Autodesk Fusion 360 part; units mm, degrees
sketch "Sketch1" plane through (0, 0, 0) normal (0, 0, 1) x (1, 0, 0)
  line L0 (284.2, -291.299) -> (-284.2, -291.299)
  line L1 (-284.2, -291.299) -> (-284.2, 291.299)
  line L2 (-284.2, 291.299) -> (284.2, 291.299)
  line L3 (284.2, 291.299) -> (284.2, -291.299)
  line L4 (284.2, -291.299) -> (-284.2, 291.299) construction
  line L5 (-284.2, -291.299) -> (284.2, 291.299) construction
  line L6 (-261.35, 291.299) -> (-261.35, -291.299) construction
  circle A0 centre (-261.35, 280.639) radius 2
  circle A1 centre (-261.35, 266.5) radius 2
  circle A2 centre (-261.35, -280.639) radius 2
  circle A3 centre (-261.35, -266.5) radius 2
  line L7 (261.35, 291.299) -> (261.35, -291.299) construction
  circle A4 centre (261.35, 280.639) radius 2
  circle A5 centre (261.35, 266.5) radius 2
  circle A6 centre (261.35, -280.639) radius 2
  circle A7 centre (261.35, -266.5) radius 2
  line L8 (-261.35, -266.5) -> (261.35, -266.5) construction
  circle A8 centre (0, -273.16) radius 2
  line L9 (0, -291.299) -> (0, 291.299) construction
  circle A9 centre (0, 273.16) radius 2
  circle A10 centre (0, 287.299) radius 2
  circle A11 centre (0, -287.299) radius 2
  line L10 (200, 225) -> (-200, 225)
  line L11 (-200, 225) -> (-200, -225)
  line L12 (-200, -225) -> (200, -225)
  line L13 (200, -225) -> (200, 225)
  line L14 (200, 225) -> (-200, -225) construction
  line L15 (-200, 225) -> (200, -225) construction
  line L16 (-289.2, 296.299) -> (289.2, 296.299)
  line L17 (289.2, 296.299) -> (289.2, -296.299)
  line L18 (289.2, -296.299) -> (-289.2, -296.299)
  line L19 (-289.2, -296.299) -> (-289.2, 296.299)
  circle A12 centre (279.2, 101.299) radius 2
  circle A13 centre (279.2, -101.299) radius 2
  circle A14 centre (-279.2, -101.299) radius 2
  circle A15 centre (-279.2, 101.299) radius 2
  line L20 (-304.8, -372.499) -> (304.8, -372.499) construction
  line L21 (304.8, -372.499) -> (304.8, 541.901) construction
  line L22 (304.8, 541.901) -> (-304.8, 541.901) construction
  line L23 (-304.8, 541.901) -> (-304.8, -372.499) construction
  line L24 (0, -372.499) -> (0, -296.299) construction
  line L25 (-261.35, 266.5) -> (261.35, 266.5) construction
  line L26 (261.35, -280.639) -> (-261.35, -280.639) construction
  line L27 (261.35, 280.639) -> (-261.35, 280.639) construction
  dimension "d1" = 568.4
  dimension "d2" = 582.598
  dimension "d3" = 22.85
  dimension "d4" = 4
  dimension "d6" = 4
  dimension "d8" = 4
  dimension "d9" = 4
  dimension "d12" = 22.85
  dimension "d13" = 4
  dimension "d14" = 4
  dimension "d17" = 4
  dimension "d18" = 4
  dimension "d21" = 4
  dimension "d22" = 4
  dimension "d23" = 4
  dimension "d24" = 4
  dimension "d28" = 450
  dimension "d29" = 400
  dimension "d30" = 5
  dimension "d31" = 5
  dimension "d32" = 5
  dimension "d33" = 5
  dimension "d37" = 4
  dimension "d38" = 4
  dimension "d39" = 4
  dimension "d40" = 4
  dimension "d41" = 190
  dimension "d42" = 190
  dimension "d43" = 5
  dimension "d44" = 5
  dimension "d45" = 190
  dimension "d46" = 190
  dimension "d47" = 5
  dimension "d49" = 5
  dimension "d51" = 609.6
  dimension "d52" = 76.2
  dimension "d53" = 914.4
  dimension "d54" = 24.799
  dimension "d55" = 24.799
  dimension "d56" = 10.66
  dimension "d57" = 10.66
  dimension "d61" = 4
  dimension "d62" = 14.139
  dimension "d63" = 14.139
  dimension "d64" = 4
extrude "Extrude1" add sketch "Sketch1" along normal blind 5 contours L0 L1 L2 L3 | L16 L17 L18 L19 makes body 1
fillet "Fillet1" radius 20 4 edges at (-200, -225, 2.5) (200, -225, 2.5) (200, 225, 2.5) (-200, 225, 2.5) on bodies 1
copy_body "Body->Comp1" bodies 1 removing the originals makes body 2 in component "Front Panel"
component "Front Panel" placed x (1, 0, 0) y (0, 1, 0) z (0, 0, 1) at (0, 0, 0)
equation "d1 = XRailLength + 218.4 mm"
equation "d2 = PrintHeight + 282.598 mm"
equation "d28 = PrintHeight + 150 mm"
equation "d29 = XRailLength + 50 mm"
equation "d30 = WallThickness"
equation "d31 = WallThickness"
equation "d32 = WallThickness"
equation "d33 = WallThickness"
equation "WallThickness = 5 mm"
equation "XRailLength = 350 mm"
equation "PrintHeight = 300 mm"
For this review, take the finished solid that the model builds, in its own axes (mm). A direction names the side the tool comes from. Give positions to 0.01 mm unless a question says otherwise; leave off trailing zeros. Order: outer loops, then holes, each group sorted by start corner. A loop starts at its lowest first (then second) coordinate and runs counter-clockwise, first axis right, second up. Notation, with made-up numbers: M 3.25,34 L 36.25,34 A16 ccw 36.25,38 Z; hole C -23.75,81.25 d9. An arc over 180 degrees is marked long. Answer in a Markdown table with one row per item. Add a question column.
(1) For faces 1 (the face through (253, 4, 0)), 2 (the face through (-193.986, 219.297, 2.535)), list the 3-axis set-ups (+Z, -Z, +X, -X, +Y, -Y) from which the entire face can be reached by the end or side of a thin tool; tool diameter is ignored.
(2) For pin 1 (3.5 mm diameter, centred on x = 0, y = 273.16, fed in from +Z), flat-tipped, find the tip position at first contact; note if it passes through.
(3) Wall thickness on probe 1 along Y at (x, z) = (0, 4.05); probe 2 along Y at (x, z) = (261.35, 3.8); probe 3 along X at (y, z) = (-266.5, 1.3): over which ranges is each line inside the solid? List them lowest first. Write a range as [from, to].
(4) Consider section C-C on z = 1.8. Give the number of separate pieces and of enclosed holes in the cut face, and give its area (3 significant figures).
(5) Mouldability with a two-part tool opening along Y and no side actions: class faces 3 (the face through (193.986, -219.297, 2.535)), 4 (the face through (253, 4, 5)) as +Y half, -Y half, draft (parallel to the pull), parting line (faces both ways), or undercut.
(6) Consider section A-A on y = 58.5. State the section outline as (x, z) points, and give its area (3 significant figures).
(7) Consider section B-B on x = 44. State the section outline as (y, z) points.
Evaluation:
| question | item | result |
|---|---|---|
| 1 | face 1 | -Z, +X, -X, +Y, -Y |
| 1 | face 2 | +Z, -Z |
| 2 | pin 1 | passes through |
| 3 | probe 1 | y = [-296.3, -289.3], [-285.3, -275.16], [-271.16, -225], [225, 271.16], [275.16, 285.3], [289.3, 296.3] |
| 3 | probe 2 | y = [-296.3, -282.64], [-278.64, -268.5], [-264.5, 264.5], [268.5, 278.64], [282.64, 296.3] |
| 3 | probe 3 | x = [-289.2, -263.35], [-259.35, 259.35], [263.35, 289.2] |
| 4 | separate pieces | 1 |
| 4 | enclosed holes | 17 |
| 4 | area | 163,000 mm^2 |
| 5 | face 3 | undercut |
| 5 | face 4 | draft |
| 6 | outline | M -289.2,0 L -200,0 L -200,5 L -289.2,5 Z; M 200,0 L 289.2,0 L 289.2,5 L 200,5 Z |
| 6 | area | 892 mm^2 |
| 7 | outline | M -296.3,0 L -225,0 L -225,5 L -296.3,5 Z; M 225,0 L 296.3,0 L 296.3,5 L 225,5 Z |
